Verification items for the finished model (mm, model axes). A direction names the side the tool comes from. Round coordinates to 2 decimals unless told otherwise and drop trailing zeros. Loops run counter-clockwise (first coordinate to the right, second up) from the corner with the lowest first, then second, coordinate; pieces in that order, holes last. Notation, with made-up numbers: M 13,80 L 64,80 A20 cw 64,89 Z; hole C 74,58.25 d11. An arc over 180 degrees is marked long. One line per item, written item: value.
from build123d import *

# Parameters (mm, degrees)
BOSS_EXTRUDE1_DEPTH = 3
SKETCH2_W           = 50
SKETCH2_H           = 20
CUT_EXTRUDE1_DEPTH  = 10


with BuildPart() as part:
    # Sketch1 → Boss-Extrude1 (new body)
    with BuildSketch(Plane.XY):
        Polygon((-32.643571906, 0), (-32.643571906, -18), (-29.643571906, -18), (-29.643571906, -28), (-32.643571906, -28), (-32.643571906, -43), (2.356428094, -43), (2.356428094, -40), (12.356428094, -40), (12.356428094, -43), (47.356428094, -43), (47.356428094, -28), (44.356428094, -28), (44.356428094, -18), (47.356428094, -18), (47.356428094, -3), (47.356428094, 0), (12.356428094, 0), (12.356428094, -3), (2.356428094, -3), (2.356428094, 0), align=None)
    extrude(amount=BOSS_EXTRUDE1_DEPTH)

    # Sketch2 → Cut-Extrude1 (cut)
    with BuildSketch(Plane.XY.offset(3)):
        with Locations((7.356428094, -23)):
            Rectangle(SKETCH2_W, SKETCH2_H)
    extrude(amount=-CUT_EXTRUDE1_DEPTH, mode=Mode.SUBTRACT)


solid = part.part
(1) Sectioned sample at B-B on x = 25. Enter the section's corners in (y, z).
Completed:
outline: M -43,0 L -33,0 L -33,3 L -43,3 Z; M -13,0 L 0,0 L 0,3 L -13,3 Z
(2) Depth check by flat-ended pin: pin 1 Ø0.9 at (y, z) = (-21, 1.5) entering from -X; pin 2 Ø1.5 at (x, z) = (10.5, 1.5) entering from -Y; pin 3 Ø1.5 at (y, z) = (-26, 1.5) entering from +X. Enter the tip coordinate at first touch or a pass-through.
Completed:
pin 1: stops at x = -29.64
pin 2: stops at y = -40
pin 3: stops at x = 44.36
(3) Sectioned sample at A-A on z = 0.5. Enter the section's corners in (x, y), and give its area (3 significant figures).
Completed:
outline: M -32.64,-43 L 2.36,-43 L 2.36,-40 L 12.36,-40 L 12.36,-43 L 47.36,-43 L 47.36,-28 L 44.36,-28 L 44.36,-18 L 47.36,-18 L 47.36,0 L 12.36,0 L 12.36,-3 L 2.36,-3 L 2.36,0 L -32.64,0 L -32.64,-18 L -29.64,-18 L -29.64,-28 L -32.64,-28 Z; hole M -17.64,-33 L 32.36,-33 L 32.36,-13 L -17.64,-13 Z
area: 2,320 mm^2
(4) Tool access check on faces 5 (the face through (47.356, -36, 1)), 6 (the face through (2.356, -42, 1)), 7 (the face through (46, -28, 1)), 8 (the face through (2.356, -2, 1)). Record the directions out of +Z, -Z, +X, -X, +Y, -Y that give a thin tool (end or side, any length) a straight path to the whole face; none if there is none.
Completed:
face 5: +Z, -Z, +X, +Y, -Y
face 6: +Z, -Z, -Y
face 7: +Z, -Z, +X
face 8: +Z, -Z, +Y
(5) Thickness scan on L1, parallel to Y at x = -4, z = 1.85; L2, parallel to X at y = -18.5, z = 1.05; L3, parallel to X at y = -29.5, z = 1. Record the ranges inside material, lowest first. Write a range as from..to.
Completed:
L1: y = -43..-33, -13..0
L2: x = -29.64..-17.64, 32.36..44.36
L3: x = -32.64..-17.64, 32.36..47.36
(6) Sectioned sample at C-C on y = -32. Enter the section's corners in (x, z).
Completed:
outline: M -32.64,0 L -17.64,0 L -17.64,3 L -32.64,3 Z; M 32.36,0 L 47.36,0 L 47.36,3 L 32.36,3 Z
(7) Mould release check, pull along X, two halves, no side actions. Record for faces 1 (the face through (30, -43, 1)), 2 (the face through (12.356, -1, 1)), 3 (the face through (-17.644, -23, 2)), 4 (the face through (-29.644, -23, 1)): +X half, -X half, draft (parallel to the pull), parting line (faces both ways), or undercut.
Completed:
face 1: draft
face 2: undercut
face 3: undercut
face 4: -X half
